Could you check a few things on this model? Use its own coordinates, in mm. Round coordinates to 2 decimals unless told otherwise and drop trailing zeros. Loops run counter-clockwise (first coordinate to the right, second up) from the corner with the lowest first, then second, coordinate; pieces in that order, holes last. Notation, with made-up numbers: (75, 87.5) -> (108, 87.5) arc R31 cw to (108, 113.5) -> close; hole circle Ø7 at (63.25, 30). An arc over 180 degrees is marked (long way). Use CSV: the item, a comma, the result in double quotes. Start each with the question number.
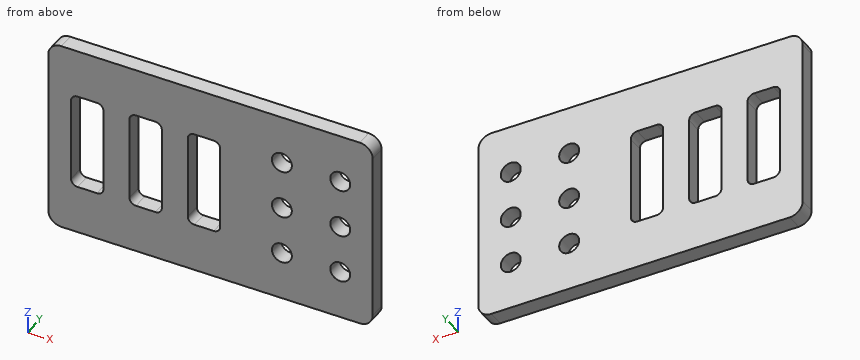
```python
from build123d import *

# Parameters (mm, degrees)
SKETCH1_W              = 100
SKETCH1_H              = 60
BOSS_EXTRUDE1_DEPTH    = 5
CUT_EXTRUDE1_START     = -6
SKETCH2_R              = 3.075
CUT_EXTRUDE1_DEPTH     = 7
SKETCH3_W              = 10
SKETCH3_H              = 30
CUT_EXTRUDE2_DEPTH     = 6
FILLET2_R              = 2
LPATTERN1_COUNT        = 3
LPATTERN1_PITCH        = 18
FILLET2_OF_LPATTERN1_R = 2
LPATTERN2_COUNT        = 2
LPATTERN2_PITCH        = 18
FILLET1_R              = 4


with BuildPart() as part:
    # Sketch1 → Boss-Extrude1 (new body)
    with BuildSketch(Plane(origin=(0, 0, 0), x_dir=(1, 0, 0), z_dir=(0, 1, 0))):
        Rectangle(SKETCH1_W, SKETCH1_H)
    extrude(amount=BOSS_EXTRUDE1_DEPTH)

    # Sketch2 → Cut-Extrude1 (cut)
    with BuildSketch(Plane(origin=(0, 5, 0), x_dir=(1, 0, 0), z_dir=(0, 1, 0)).offset(CUT_EXTRUDE1_START)):
        with Locations((40, 15)):
            Circle(SKETCH2_R)
        with Locations((40, -15)):
            Circle(SKETCH2_R)
        with Locations((40, 0)):
            Circle(SKETCH2_R)
    cut_extrude1 = extrude(amount=CUT_EXTRUDE1_DEPTH, mode=Mode.SUBTRACT)

    # Sketch3 → Cut-Extrude2 (cut, through all)
    with BuildSketch(Plane(origin=(0, 5, 0), x_dir=(1, 0, 0), z_dir=(0, 1, 0))):
        with Locations((-38, 0)):
            Rectangle(SKETCH3_W, SKETCH3_H)
    cut_extrude2 = extrude(amount=-CUT_EXTRUDE2_DEPTH, mode=Mode.SUBTRACT)

    # Fillet2
    fillet2_edges = [part.edges().sort_by_distance(p)[0] for p in [
        (-33, 2.5, -15),
        (-33, 2.5, 15),
        (-43, 2.5, 15),
        (-43, 2.5, -15),
    ]]
    fillet(fillet2_edges, radius=FILLET2_R)

    # LPattern1: Cut-Extrude2 ×3
    with Locations(*[(i * LPATTERN1_PITCH, 0, 0) for i in range(1, LPATTERN1_COUNT)]):
        add(cut_extrude2, mode=Mode.SUBTRACT)

    # Fillet2 of LPattern1
    fillet2_of_lpattern1_edges = [part.edges().sort_by_distance(p)[0] for p in [
        (-15, 2.5, -15),
        (-15, 2.5, 15),
        (-25, 2.5, 15),
        (-25, 2.5, -15),
        (3, 2.5, -15),
        (3, 2.5, 15),
        (-7, 2.5, 15),
        (-7, 2.5, -15),
    ]]
    fillet(fillet2_of_lpattern1_edges, radius=FILLET2_OF_LPATTERN1_R)

    # LPattern2: Cut-Extrude1 ×2
    with Locations(*[(-i * LPATTERN2_PITCH, 0, 0) for i in range(1, LPATTERN2_COUNT)]):
        add(cut_extrude1, mode=Mode.SUBTRACT)

    # Fillet1
    fillet1_edges = [part.edges().sort_by_distance(p)[0] for p in [
        (50, 2.5, 30),
        (-50, 2.5, 30),
        (-50, 2.5, -30),
        (50, 2.5, -30),
    ]]
    fillet(fillet1_edges, radius=FILLET1_R)


solid = part.part
```
1. Will these pins go through, and if not, where does the flat tip stop? pin 1 (8 mm diameter, centred on x = -20.5, z = 2, fed in from -Y); pin 2 (10 mm diameter, centred on x = 34, z = 15.5, fed in from -Y).
2. Suppose I cut it at D-D (y = 2.6). State how many separate pieces and enclosed holes the cut face has, then the cut area to 3 significant figures.
3. Suppose I cut it at A-A (x = 40). List the corners of the cut face in (y, z) for me (3 decimals).
4. If I drill on L1, parallel to X at y = 4, z = 10.5; L2, parallel to Z at x = 22, y = 2.85 (3 decimals); L3, parallel to Z at x = -17.5, y = 1.6, over which ranges is the centre line in solid material (lowest first)?
5. Suppose I cut it at B-B (z = 7). List the corners of the cut face in (x, y) for me, then the cut area to 3 significant figures.
6. Suppose I cut it at C-C (z = 0). List the corners of the cut face in (x, y) for me (3 decimals), then the cut area to 4 significant figures.
Geometry check:
1,pin 1,"passes through"
1,pin 2,"stops at y = 0"
2,separate pieces,"1"
2,enclosed holes,"9"
2,area,"4,920 mm²"
3,outline,"(0, -30) -> (5, -30) -> (5, -18.075) -> (0, -18.075) -> close; (0, -11.925) -> (5, -11.925) -> (5, -3.075) -> (0, -3.075) -> close; (0, 3.075) -> (5, 3.075) -> (5, 11.925) -> (0, 11.925) -> close; (0, 18.075) -> (5, 18.075) -> (5, 30) -> (0, 30) -> close"
4,L1,"x = -50 to -43, -33 to -25, -15 to -7, 3 to 50"
4,L2,"z = -30 to -18.075, -11.925 to -3.075, 3.075 to 11.925, 18.075 to 30"
4,L3,"z = -30 to -15, 15 to 30"
5,outline,"(-50, 0) -> (-43, 0) -> (-43, 5) -> (-50, 5) -> close; (-33, 0) -> (-25, 0) -> (-25, 5) -> (-33, 5) -> close; (-15, 0) -> (-7, 0) -> (-7, 5) -> (-15, 5) -> close; (3, 0) -> (50, 0) -> (50, 5) -> (3, 5) -> close"
5,area,"350 mm²"
6,outline,"(-50, 0) -> (-43, 0) -> (-43, 5) -> (-50, 5) -> close; (-33, 0) -> (-25, 0) -> (-25, 5) -> (-33, 5) -> close; (-15, 0) -> (-7, 0) -> (-7, 5) -> (-15, 5) -> close; (3, 0) -> (18.925, 0) -> (18.925, 5) -> (3, 5) -> close; (25.075, 0) -> (36.925, 0) -> (36.925, 5) -> (25.075, 5) -> close; (43.075, 0) -> (50, 0) -> (50, 5) -> (43.075, 5) -> close"
6,area,"288.5 mm²"
